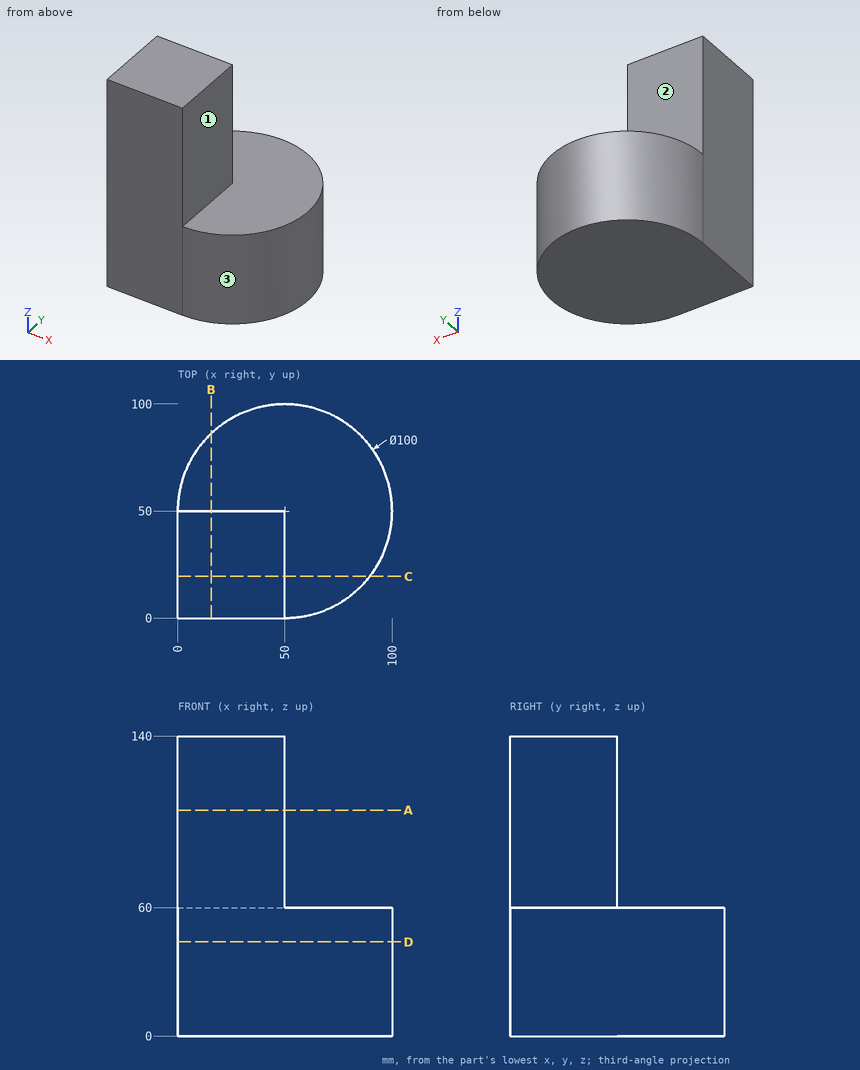
Job drawing, mm, ordinate dimensions from the low corner. One solid piece. A direction names the side the tool comes from. Round coordinates to 2 decimals unless told otherwise and drop trailing zeros. Loops run counter-clockwise (first coordinate to the right, second up) from the corner with the lowest first, then second, coordinate; pieces in that order, holes last.
(1) Wall check: line 1 along X through (y, z) = (44, 113.5); line 2 along Z through (x, y) = (47.5, 85.5). Give the ranges that are in metal, low to high.
(2) Cut at D-D (z = 44). Give the cut face in (x, y).
(3) Drop flat-ended pins along their axis: pin 1 (10 mm diameter, centred on x = 55.5, z = 47, fed in from +Y); pin 2 (1.5 mm diameter, centred on x = 75, z = 51.5, fed in from -Y); pin 3 (25 mm diameter, centred on x = 17.5, z = 93, fed in from +Y). Give the stop position or say it passes through.
(4) Cut at A-A (z = 105.5). Give the cut face in (x, y), plus the area to 3 significant figures.
(5) Cut at C-C (y = 19.5). Give the cut face in (x, z), plus the area to 3 significant figures.
(6) Which spindle directions (+Z, -Z, +X, -X, +Y, -Y) get a long thin tool onto all of the face, cutting with end or side? Do the marked faces 1, 2 and 3. Say none if no direction does.
(7) Cut at B-B (x = 15.5). Give the cut face in (y, z), plus the area to 3 significant figures.
Findings below:
1. line 1: x = 0 to 50
1. line 2: z = 0 to 60
2. outline: (0, 0) - (50, 0) arc R50 ccw (long way) to (0, 50) - close
3. pin 1: stops at y = 100
3. pin 2: stops at y = 6.27
3. pin 3: stops at y = 50
4. outline: (0, 0) - (50, 0) - (50, 50) - (0, 50) - close
4. area: 2,500 mm2
5. outline: (0, 0) - (89.62, 0) - (89.62, 60) - (50, 60) - (50, 140) - (0, 140) - close
5. area: 9,380 mm2
6. face 1: +Z, +X, +Y, -Y
6. face 2: +Z, +X, -X, +Y
6. face 3: +Z, -Z
7. outline: (0, 0) - (86.19, 0) - (86.19, 60) - (50, 60) - (50, 140) - (0, 140) - close
7. area: 9,170 mm2
